Job drawing, mm, ordinate dimensions from the low corner. One solid piece. A direction names the side the tool comes from. Coordinates: 2 decimals unless noted, no trailing zeros. Order: outer loops, then holes, each group sorted by start corner. A loop starts at its lowest first (then second) coordinate and runs counter-clockwise, first axis right, second up. Notation, with made-up numbers: M 1,42 L 27,42 A22 ccw 27,79 Z; hole C 46.5,-22 d4. An arc over 180 degrees is marked long. Write item = value, one per line.
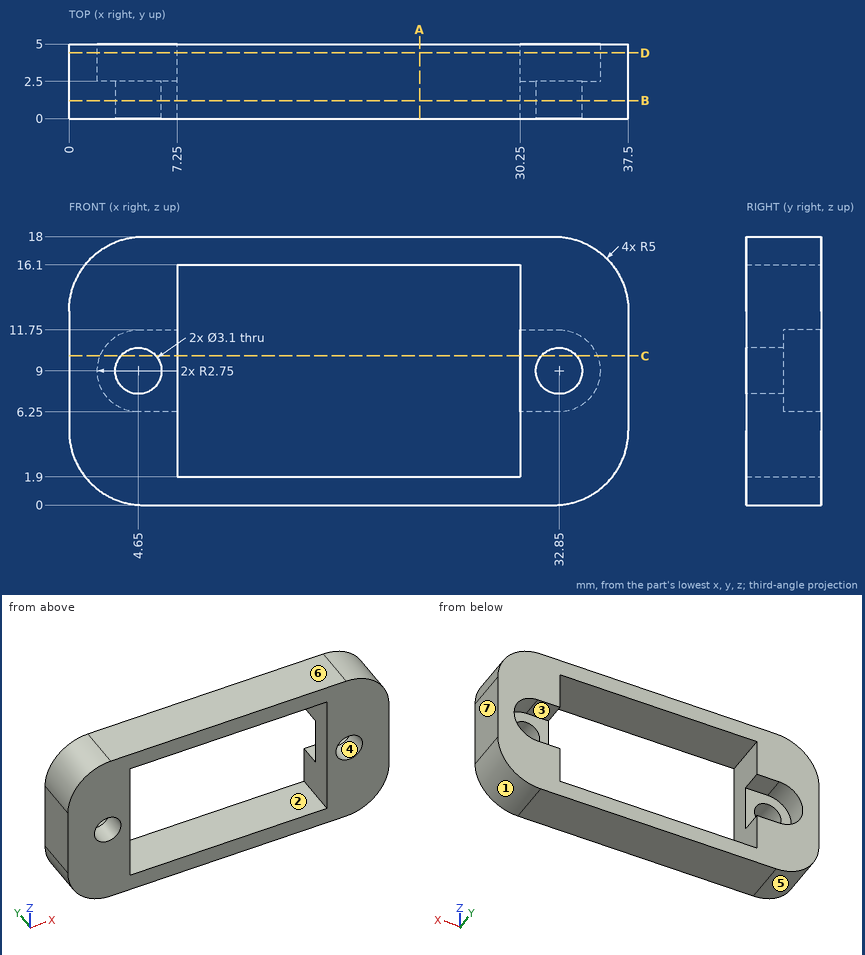
(1) Tool access for the marked faces 1, 2 and 3: list every direction of +Z, -Z, +X, -X, +Y, -Y with a clear straight run to the whole face (end or side of a thin tool).
Evaluation:
face_1 = -Z, +X, +Y, -Y
face_2 = +Y, -Y
face_3 = +Y
(2) Pin check, flat tips, straight feed: pin 1 Ø1.6 at (x, z) = (34, 10) entering from +Y; pin 2 Ø3 at (x, z) = (9, 10.5) entering from +Y. Stop position of each tip, or through.
Evaluation:
pin_1 = 2.5
pin_2 = through
(3) Pull direction X, two halves, no side cores. Call the marked faces 4, 5, 6 and 7: +X half, -X half, draft (parallel to the pull), parting line (faces both ways), or undercut.
Evaluation:
face_4 = undercut
face_5 = -X half
face_6 = draft
face_7 = +X half
(4) Wall check: line 1 (X direction, y = 1.6, z = 9); line 2 (Z direction, x = 14.5, y = 3.95); line 3 (Z direction, x = 5, y = 2.85). Give the ranges that are in metal, low to high. Write a range as from..to.
Evaluation:
line_1 = 0..3.1, 6.2..7.25, 30.25..31.3, 34.4..37.5
line_2 = 0..1.9, 16.1..18
line_3 = 0..6.25, 11.75..18
(5) Slice it at B-B, the plane y = 1.2. Write the cut outline in (x, z).
Evaluation:
outline = M 0,5 A5 ccw 5,0 L 32.5,0 A5 ccw 37.5,5 L 37.5,13 A5 ccw 32.5,18 L 5,18 A5 ccw 0,13 Z; hole C 4.65,9 d3.1; hole M 7.25,1.9 L 30.25,1.9 L 30.25,16.1 L 7.25,16.1 Z; hole C 32.85,9 d3.1
(6) Slice it at A-A, the plane x = 23.5. Write the cut outline in (y, z), then the cut area to 3 significant figures.
Evaluation:
outline = M 0,0 L 5,0 L 5,1.9 L 0,1.9 Z; M 0,16.1 L 5,16.1 L 5,18 L 0,18 Z
area = 19.0 mm²
(7) Slice it at D-D, the plane y = 4.4. Write the cut outline in (x, z).
Evaluation:
outline = M 0,5 A5 ccw 5,0 L 32.5,0 A5 ccw 37.5,5 L 37.5,13 A5 ccw 32.5,18 L 5,18 A5 ccw 0,13 Z; hole M 4.65,6.25 L 7.25,6.25 L 7.25,1.9 L 30.25,1.9 L 30.25,6.25 L 32.85,6.25 A2.75 ccw 32.85,11.75 L 30.25,11.75 L 30.25,16.1 L 7.25,16.1 L 7.25,11.75 L 4.65,11.75 A2.75 ccw Z
(8) Slice it at C-C, the plane z = 10. Write the cut outline in (x, y), then the cut area to 3 significant figures.
Evaluation:
outline = M 0,0 L 3.47,0 L 3.47,2.5 L 2.09,2.5 L 2.09,5 L 0,5 Z; M 5.83,0 L 7.25,0 L 7.25,2.5 L 5.83,2.5 Z; M 30.25,0 L 31.67,0 L 31.67,2.5 L 30.25,2.5 Z; M 34.03,0 L 37.5,0 L 37.5,5 L 35.41,5 L 35.41,2.5 L 34.03,2.5 Z
area = 34.8 mm²
